from build123d import *

# Parameters (mm, degrees)
F0_W        = 186.3179504871
F0_H        = 91.0190269351
F1_DEPTH    = 60
F3_DEPTH    = 25
F5_DEPTH    = 25
F7_DEPTH    = 181
F10_D       = 30
F10_ON_F9_D = 30


with BuildPart() as f1:
    # F0 (on Front) → F1 (new body, symmetric)
    with BuildSketch(Plane.XZ):
        with Locations((0.5706548691, -4.2798891664)):
            Rectangle(F0_W, F0_H)
    extrude(amount=F1_DEPTH, both=True)

    # F2 (on face) → F3 (join)
    with BuildSketch(Plane.XZ.offset(60)):
        with BuildLine():
            ThreePointArc((37.2350551188, 41.2296243012), (-1.3436250294, 22.7301151194), (-39.9223051776, 41.2296243012))
            Line((-39.9223051776, 41.2296243012), (-54.8638885904, 41.2296243012))
            ThreePointArc((-54.8638885904, 41.2296243012), (-0.9986385703, 11.1155049194), (52.8666114498, 41.2296243012))
            Line((52.8666114498, 41.2296243012), (37.2350551188, 41.2296243012))
        make_face()
    extrude(amount=F3_DEPTH)

    # F4 (on face) → F5 (join)
    with BuildSketch(Plane(origin=(0, 60, 0), x_dir=(-1, 0, 0), z_dir=(0, 1, 0))):
        with BuildLine():
            Line((-36.6474762559, 41.2296243012), (-55.402355561, 41.2296243012))
            ThreePointArc((-55.402355561, 41.2296243012), (1.44476071, 10.6097235864), (58.291876981, 41.2296243012))
            Line((58.291876981, 41.2296243012), (40.3841994703, 41.2296243012))
            ThreePointArc((40.3841994703, 41.2296243012), (1.8683616072, 21.7640944123), (-36.6474762559, 41.2296243012))
        make_face()
    extrude(amount=F5_DEPTH)

    # F7 (cut): a face of the model
    f7_faces = [f1.faces().sort_by_distance(p)[0] for p in [
        (-1.3436250294, -60, 33.6967312772),
    ]]
    extrude(f7_faces, amount=-F7_DEPTH, mode=Mode.SUBTRACT)

    # F10 (through all)
    with Locations(Plane.XY.offset(41.2296243012)):
        with Locations((-72.9959234595, 0)):
            Hole(F10_D / 2)

    # F10 on F9 (through all)
    with Locations(Plane.XY.offset(41.2296243012)):
        with Locations((74.4606032968, 0)):
            Hole(F10_ON_F9_D / 2)


solid = f1.part
Here's how the part is built. I have some questions about the finished solid (model axes, mm). A direction names the side the tool comes from. Coordinates: 2 decimals unless noted, no trailing zeros. Order: outer loops, then holes, each group sorted by start corner. A loop starts at its lowest first (then second) coordinate and runs counter-clockwise, first axis right, second up. Notation, with made-up numbers: M 28,30.25 L 76,30.25 A17 ccw 76,62.25 Z; hole C 38.5,20 d10. An arc over 180 degrees is marked long. Answer as CSV lines item,"result".
Item 1: On a 3-axis mill with a long thin cutter (end or side, diameter ignored), from which of +Z, -Z, +X, -X, +Y, -Y can I reach the whole of each face in a straight line? I mean faces 1 (the face through (-7.36, 72.32, 22.08)), 2 (the face through (-1.9, -72.32, 11.12)), 3 (the face through (-0.503, 72.325, 10.616)). Say none if no direction works.
Results found:
face 1,"+Z, +Y"
face 2,"-Z, -Y"
face 3,"-Z, +Y"
Item 2: We'd pull the mould along X, two halves only. Please class faces 4 (the face through (93.73, -1, -5)), 5 (the face through (-58.01, 0.66, -4.92)), 6 (the face through (-1, -1, -49.789)), 7 (the face through (-13.2, 60, 23.6)): +X half, -X half, draft (parallel to the pull), parting line (faces both ways), or undercut.
Results found:
face 4,"+X half"
face 5,"undercut"
face 6,"draft"
face 7,"undercut"
Item 3: Imagine slicing it at D-D on z = 5.5. Write out the boundary of the cut face in (x, y), plus the area to 3 significant figures.
Results found:
outline,"M -92.59,-60 L 93.73,-60 L 93.73,60 L -92.59,60 Z; hole C -73,0 d30; hole C 74.46,0 d30"
area,"20,900 mm2"
Item 4: Imagine slicing it at B-B on z = 31. Write out the boundary of the cut face in (x, y), plus the area to 3 significant figures.
Results found:
outline,"M -92.59,-60 L -47.03,-60 L -47.03,-85 L -28.73,-85 L -28.73,60 L -30.12,60 L -30.12,85 L -50.03,85 L -50.03,60 L -92.59,60 Z; M 26.04,-85 L 45.04,-85 L 45.04,-60 L 93.73,-60 L 93.73,60 L 47.14,60 L 47.14,85 L 26.39,85 L 26.39,60 L 26.04,60 Z; hole C -73,0 d30; hole C 74.46,0 d30"
area,"16,300 mm2"
Item 5: Imagine slicing it at C-C on x = 64. Write out the boundary of the cut face in (y, z), plus the area to 3 significant figures.
Results found:
outline,"M -60,-49.79 L -10.75,-49.79 L -10.75,41.23 L -60,41.23 Z; M 10.75,-49.79 L 60,-49.79 L 60,41.23 L 10.75,41.23 Z"
area,"8,970 mm2"
Item 6: For pin 1 (18 mm diameter, centred on x = -73, y = 0, fed in from +Z); pin 2 (1.5 mm diameter, centred on x = 3, z = -7, fed in from -Y), each with a flat end and sliding along its axis, tell me the tip position at first contact or that it passes through.
Results found:
pin 1,"through"
pin 2,"y = -60"
Item 7: Imagine slicing it at A-A on y = 0. Write out the boundary of the cut face in (x, z).
Results found:
outline,"M -92.59,-49.79 L -88,-49.79 L -88,41.23 L -92.59,41.23 Z; M -58,-49.79 L 59.46,-49.79 L 59.46,41.23 L 37.24,41.23 A49.48 cw -39.92,41.23 L -58,41.23 Z; M 89.46,-49.79 L 93.73,-49.79 L 93.73,41.23 L 89.46,41.23 Z"
Item 8: If I drill on line 1 (Y direction, x = 73.5, z = 3); line 2 (X direction, y = -11, z = 27.5); line 3 (Y direction, x = -26.5, z = -31), over which ranges is the centre line in solid material (lowest first)?
Results found:
line 1,"-60 to -14.97, 14.97 to 60"
line 2,"-92.59 to -83.19, -62.8 to -22.54, 19.85 to 64.26, 84.66 to 93.73"
line 3,"-60 to 60"
